For this review, take the finished solid that the model builds, in its own axes (mm). A direction names the side the tool comes from. Coordinates: 2 decimals unless noted, no trailing zeros. Write each loop counter-clockwise with the first axis right and the second up, starting at its lowest first coordinate (ties: lowest second). Pieces come first, ordered by that corner, then holes. Notation, with made-up numbers: (73.25, -39.75) - (115.25, -39.75) arc R30 ccw to (115.25, -17.75) - close; hole circle Ø10 at (56.25, 19). An arc over 180 degrees is marked (long way). Use one line per item in the form item = value. Start each with the question number.
1) For L1, parallel to Y at x = 23, z = -3.1; L2, parallel to Z at x = 28, y = 117.2; L3, parallel to X at y = 46, z = -70, list the stretches that pass through material, from the lowest coordinate up. Write a range as from..to.
2) Insertion check: P1, Ø4, axis at y = 23, z = -45.5, coming from the +X side; P2, Ø2.5, axis at x = 14.5, y = 117.5, coming from the +Z side; P3, Ø6.5, axis at x = 28, z = -105, coming from the -Y side. Each pin has a flat end and moves straight along its axis. Give the tip position at first contact, or say it passes through.
3) We need section B-B (x = 23). Give the boundary of the cut face in (y, z) (3 decimals), plus the area to 3 significant figures.
4) We need section D-D (z = -57.5). Give the boundary of the cut face in (x, y), plus the area to 3 significant figures.
5) Mouldability with a two-part tool opening along X and no side actions: class faces 4 (the cylindrical face through (2, 20, -1)), 5 (the flat face through (20, 18, -5)), 6 (the cylindrical face through (-17.3, 2.82, -112.95)) as pulls with the +X half, pulls with the -X half, needs draft (parallel to the pull), parting line crosses it, or undercut.
6) We need section C-C (z = -10). Give the boundary of the cut face in (x, y).
7) Tool access review of faces 1 (the cylindrical face through (39, 117, -118)), 2 (the flat face through (20, 117, -90)), 3 (the flat face through (0, 49, -74)): name each direction out of +Z, -Z, +X, -X, +Y, -Y from which nothing blocks a thin tool from reaching the whole face with its end or side.
8) We need section A-A (y = 19). Give the boundary of the cut face in (x, z) (3 decimals).
```python
from build123d import *

# Parameters (mm, degrees)
ESTRUSIONE_ESTRUSIONE1_DEPTH    = 5
SCHIZZO2_W                      = 120
SCHIZZO2_H                      = 5.571316046
ESTRUSIONE_ESTRUSIONE2_DEPTH    = 30
SCHIZZO3_W                      = 5
SCHIZZO3_H                      = 23
ESTRUSIONE_ESTRUSIONE3_DEPTH    = 30
SCHIZZO4_W                      = 30
SCHIZZO4_H                      = 5
ESTRUSIONE_ESTRUSIONE4_DEPTH    = 35
RACCORDO1_R                     = 5
FORO_FILETTATO_M6_2_D           = 5
FORO_FILETTATO_M6_2_CSINK_D     = 6.05
FORO_FILETTATO_M6_2_CSINK_ANGLE = 90
FORO_FILETTATO_M6_3_D           = 5
FORO_FILETTATO_M6_3_CSINK_D     = 6.05
FORO_FILETTATO_M6_3_CSINK_ANGLE = 90
SCHIZZO13_R                     = 4
TAGLIO_ESTRUSIONE1_DEPTH        = 171.569410245


with BuildPart() as part:
    # Schizzo1 → Estrusione-Estrusione1 (new body)
    with BuildSketch(Plane(origin=(0, 0, 0), x_dir=(0, 0, -1), z_dir=(1, 0, 0))):
        Polygon((0, 0), (120, 0), (120, 120), (90, 120), (0, 30), align=None)
    extrude(amount=ESTRUSIONE_ESTRUSIONE1_DEPTH)

    # Schizzo2 → Estrusione-Estrusione2 (add)
    with BuildSketch(Plane.ZY):
        with Locations((-60, 2.785658023)):
            Rectangle(SCHIZZO2_W, SCHIZZO2_H)
    extrude(amount=ESTRUSIONE_ESTRUSIONE2_DEPTH)

    # Schizzo3 → Estrusione-Estrusione3 (add)
    with BuildSketch(Plane(origin=(5, 0, 0), x_dir=(0, 0, -1), z_dir=(1, 0, 0))):
        with Locations((2.5, 18.5)):
            Rectangle(SCHIZZO3_W, SCHIZZO3_H)
    extrude(amount=ESTRUSIONE_ESTRUSIONE3_DEPTH)

    # Schizzo4 → Estrusione-Estrusione4 (add)
    with BuildSketch(Plane(origin=(5, 0, 0), x_dir=(0, 0, -1), z_dir=(1, 0, 0))):
        with Locations((105, 117.5)):
            Rectangle(SCHIZZO4_W, SCHIZZO4_H)
    extrude(amount=ESTRUSIONE_ESTRUSIONE4_DEPTH)

    # Raccordo1
    # the kernel refuses this fillet: 5 mm, written as the material it takes off along each edge
    with BuildSketch(Plane(origin=(40, 102.5, -120), x_dir=(0, 0, 1), z_dir=(0, 1, 0)), Plane(origin=(35, 7, 12.5), x_dir=(0, 1, 0), z_dir=(0, 0, -1))) as raccordo1_piece_1:
        with BuildLine():
            CenterArc((RACCORDO1_R, -RACCORDO1_R), RACCORDO1_R, 90, 90)
            Line((0, -RACCORDO1_R), (0, 0))
            Line((0, 0), (RACCORDO1_R, 0))
        make_face()
    extrude(amount=30, mode=Mode.SUBTRACT)
    with BuildSketch(Plane(origin=(40, 132.5, -90), x_dir=(-1, 0, 0), z_dir=(0, -1, 0)), Plane(origin=(35, 30, -17.5), x_dir=(-1, 0, 0), z_dir=(0, 0, 1))) as raccordo1_piece_2:
        with BuildLine():
            CenterArc((RACCORDO1_R, RACCORDO1_R), RACCORDO1_R, 180, 90)
            Line((0, RACCORDO1_R), (0, 0))
            Line((0, 0), (RACCORDO1_R, 0))
        make_face()
    extrude(amount=30, mode=Mode.SUBTRACT)
    with BuildSketch(Plane(origin=(-30, 18.071316046, 0), x_dir=(0, 0, -1), z_dir=(0, -1, 0)), Plane(origin=(-30, -12.5, -120), x_dir=(0, 0, 1), z_dir=(0, 1, 0))) as raccordo1_piece_3:
        with BuildLine():
            CenterArc((RACCORDO1_R, RACCORDO1_R), RACCORDO1_R, 180, 90)
            Line((0, RACCORDO1_R), (0, 0))
            Line((0, 0), (RACCORDO1_R, 0))
        make_face()
    extrude(amount=30.571316046, mode=Mode.SUBTRACT)
    with BuildSketch(Plane(origin=(5, 0, 12.5), x_dir=(-1, 0, 0), z_dir=(0, 0, -1))) as raccordo1_piece_4:
        with BuildLine():
            CenterArc((RACCORDO1_R, RACCORDO1_R), RACCORDO1_R, 180, 90)
            Line((0, RACCORDO1_R), (0, 0))
            Line((0, 0), (RACCORDO1_R, 0))
        make_face()
    extrude(amount=145, mode=Mode.SUBTRACT)
    with BuildSketch(Plane(origin=(0, 120, -132.5), x_dir=(0, -1, 0), z_dir=(0, 0, 1))) as raccordo1_piece_5:
        with BuildLine():
            CenterArc((RACCORDO1_R, RACCORDO1_R), RACCORDO1_R, 180, 90)
            Line((0, RACCORDO1_R), (0, 0))
            Line((0, 0), (RACCORDO1_R, 0))
        make_face()
    extrude(amount=55, mode=Mode.SUBTRACT)
    with BuildSketch(Plane(origin=(0, 42.5, 0), x_dir=(0, 0, -1), z_dir=(0, -1, 0))) as raccordo1_piece_6:
        with BuildLine():
            CenterArc((RACCORDO1_R, RACCORDO1_R), RACCORDO1_R, 180, 90)
            Line((0, RACCORDO1_R), (0, 0))
            Line((0, 0), (RACCORDO1_R, 0))
        make_face()
    extrude(amount=36.928683954, mode=Mode.SUBTRACT)

    # Foro filettato M6-2 (through all)
    with Locations(Plane(origin=(0, 120, 0), x_dir=(1, 0, 0), z_dir=(0, 1, 0))):
        with Locations((28, 105)):
            CounterSinkHole(FORO_FILETTATO_M6_2_D / 2, FORO_FILETTATO_M6_2_CSINK_D / 2, counter_sink_angle=FORO_FILETTATO_M6_2_CSINK_ANGLE)

    # Foro filettato M6-3 (through all)
    with Locations(Plane.XY):
        with Locations((23, 19)):
            CounterSinkHole(FORO_FILETTATO_M6_3_D / 2, FORO_FILETTATO_M6_3_CSINK_D / 2, counter_sink_angle=FORO_FILETTATO_M6_3_CSINK_ANGLE)

    # Schizzo13 → Taglio-Estrusione1 (cut, through all)
    with BuildSketch(Plane(origin=(0, 5.571316046, 0), x_dir=(1, 0, 0), z_dir=(0, 1, 0))):
        with Locations(Location((-20, 110, 0), (0, 0, 270))):
            Circle(SCHIZZO13_R)
        with Locations(Location((-20, 10, 0), (0, 0, 270))):
            Circle(SCHIZZO13_R)
    extrude(amount=-TAGLIO_ESTRUSIONE1_DEPTH, mode=Mode.SUBTRACT)


solid = part.part
```
Determined:
q1.L1 = 7..16.5, 21.5..30
q1.L2 = -120..-107.5, -102.5..-90
q1.L3 = 0..5
q2.P1 = 5
q2.P2 = -90
q2.P3 = 115
q3.outline = (7, -5) - (16.5, -5) - (16.5, -0.525) - (15.975, 0) - (7, 0) - close; (21.5, -5) - (30, -5) - (30, 0) - (22.025, 0) - (21.5, -0.525) - close; (115, -120) - (120, -120) - (120, -90) - (115, -90) - close
q3.area = 240 mm²
q4.outline = (-30, 0) - (0, 0) arc R5 ccw to (5, 5) - (5, 87.5) - (0, 87.5) - (0, 5.57) - (-30, 5.57) - close
q4.area = 599 mm²
q5.face_4 = pulls with the -X half
q5.face_5 = needs draft
q5.face_6 = undercut
q6.outline = (-30, 0) - (-24, 0) - (-24, 5.57) - (-30, 5.57) - close; (-16, 0) - (0, 0) arc R5 ccw to (5, 5) - (5, 40) - (0, 40) - (0, 5.57) - (-16, 5.57) - close
q7.face_1 = -Z, +X, +Y, -Y
q7.face_2 = +Z, +X, +Y, -Y
q7.face_3 = +Z, -Z, -X, +Y
q8.outline = (0, -120) - (5, -120) - (5, -5) - (20.5, -5) - (20.5, -0.525) - (19.975, 0) - (5, 0) arc R5 ccw to (0, -5) - close; (25.5, -5) - (35, -5) - (35, 0) - (26.025, 0) - (25.5, -0.525) - close
